Geometry: final body of the model. Coordinates: model frame, mm. Round coordinates to 2 decimals unless told otherwise and drop trailing zeros. Order: outer loops, then holes, each group sorted by start corner. A loop starts at its lowest first (then second) coordinate and runs counter-clockwise, first axis right, second up. Notation, with made-up numbers: M -5.75,22.25 L 52.25,22.25 A29 cw 52.25,45.25 Z; hole C 82.5,-12.75 d10. An arc over 180 degrees is marked long. Return JSON: item names as keys, results as strings. Group by question number.
Q1. Cut plane A-A on y = 10. Output: boundary loops of the cut face in (x, z), and give its area (3 significant figures).
Q2. Ray query, probe 1 along Y at (x, z) = (99, 1.9); probe 2 along Y at (x, z) = (67, 1.8); probe 3 along X at (y, z) = (46, 4). Return the intervals inside material, ascending.
Q3. Cut plane C-C on z = 3.85. Count the separate pieces of the cut face and the enclosed holes in it, and give its area (3 significant figures).
Q4. Cut plane B-B on x = 3. Output: boundary loops of the cut face in (y, z).
Q5. Cut plane D-D on x = 22.5. Output: boundary loops of the cut face in (y, z).
Q6. Contact query for flat-ended pins moving along their axis: pin 1 (5 mm diameter, centred on x = 99, y = 10, fed in from -Z); pin 2 (3 mm diameter, centred on x = 12.5, y = 44.5, fed in from +Z). Output: stop coordinate, or through.
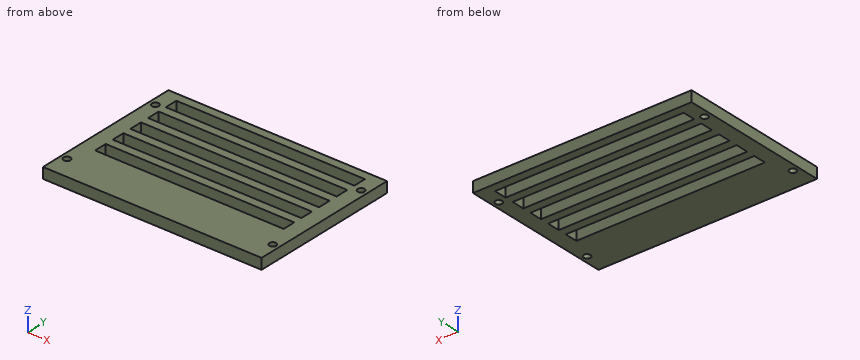
```python
from build123d import *

# Parameters (mm, degrees)
SKETCH_1_W             = 102
SKETCH_1_H             = 65
EXTRUDE_1_DEPTH        = 5
SKETCH_2_R             = 1.6
CUT_EXTRUDE_1_DEPTH    = 122.053707089
SKETCH_3_W             = 102
SKETCH_3_H             = 6
EXTRUDE_2_DEPTH        = 5
SKETCH_4_W             = 88
SKETCH_4_H             = 6
CUT_EXTRUDE_2_DEPTH    = 125.378454726
PATTERN_LINEAR_1_COUNT = 5
PATTERN_LINEAR_1_PITCH = 10


with BuildPart() as part:
    # 草图1 → 凸台-拉伸1 (new body)
    with BuildSketch(Plane.XY):
        with Locations((51, 32.5)):
            Rectangle(SKETCH_1_W, SKETCH_1_H)
    extrude(amount=EXTRUDE_1_DEPTH)

    # 草图2 → 切除-拉伸1 (cut, through all)
    with BuildSketch(Plane.XY.offset(5)):
        with Locations((3, 60)):
            Circle(SKETCH_2_R)
        with Locations((99, 10)):
            Circle(SKETCH_2_R)
        with Locations((3, 10)):
            Circle(SKETCH_2_R)
        with Locations((99, 60)):
            Circle(SKETCH_2_R)
    extrude(amount=-CUT_EXTRUDE_1_DEPTH, mode=Mode.SUBTRACT)

    # 草图3 → 凸台-拉伸2 (add)
    with BuildSketch(Plane.XY.offset(5)):
        with Locations((51, 68)):
            Rectangle(SKETCH_3_W, SKETCH_3_H)
    extrude(amount=-EXTRUDE_2_DEPTH)

    # 草图4 → 切除-拉伸2 (cut, through all)
    with BuildSketch(Plane.XY.offset(5)):
        with Locations((51, 64)):
            Rectangle(SKETCH_4_W, SKETCH_4_H)
    cut_extrude_2 = extrude(amount=-CUT_EXTRUDE_2_DEPTH, mode=Mode.SUBTRACT)

    # 阵列(线性)1: 切除-拉伸2 ×5
    with Locations(*[(0, -i * PATTERN_LINEAR_1_PITCH, 0) for i in range(1, PATTERN_LINEAR_1_COUNT)]):
        add(cut_extrude_2, mode=Mode.SUBTRACT)


solid = part.part
```
Result sheet:
{
 "1": {"outline": "M 0,0 L 1.4,0 L 1.4,5 L 0,5 Z; M 4.6,0 L 97.4,0 L 97.4,5 L 4.6,5 Z; M 100.6,0 L 102,0 L 102,5 L 100.6,5 Z", "area": "478 mm²"},
 "2": {"probe 1": "y = 0 to 8.4, 11.6 to 58.4, 61.6 to 71", "probe 2": "y = 0 to 21, 27 to 31, 37 to 41, 47 to 51, 57 to 61, 67 to 71", "probe 3": "x = 0 to 7, 95 to 102"},
 "3": {"separate pieces": "1", "enclosed holes": "9", "area": "4,570 mm²"},
 "4": {"outline": "M 0,0 L 8.4,0 L 8.4,5 L 0,5 Z; M 11.6,0 L 58.4,0 L 58.4,5 L 11.6,5 Z; M 61.6,0 L 71,0 L 71,5 L 61.6,5 Z"},
 "5": {"outline": "M 0,0 L 21,0 L 21,5 L 0,5 Z; M 27,0 L 31,0 L 31,5 L 27,5 Z; M 37,0 L 41,0 L 41,5 L 37,5 Z; M 47,0 L 51,0 L 51,5 L 47,5 Z; M 57,0 L 61,0 L 61,5 L 57,5 Z; M 67,0 L 71,0 L 71,5 L 67,5 Z"},
 "6": {"pin 1": "stops at z = 0", "pin 2": "passes through"}
}
